Check sheet for the modelled part. Datum: model origin and axes. Units: mm. Coordinates: 2 decimals unless noted, no trailing zeros. Order: outer loops, then holes, each group sorted by start corner. A loop starts at its lowest first (then second) coordinate and runs counter-clockwise, first axis right, second up.
from build123d import *

# Parameters (mm, degrees)
SKETCH1_R           = 1.5
BOSS_EXTRUDE1_DEPTH = 3.18
SKETCH2_R           = 10
CUT_EXTRUDE1_DEPTH  = 3.18


with BuildPart() as part:
    # Sketch1 → Boss-Extrude1 (new body)
    with BuildSketch(Plane(origin=(0, 0, 0), x_dir=(1, 0, 0), z_dir=(0, 1, 0))):
        with BuildLine():
            Line((-36.950288588, 11.035836474), (7.707885855, 14.942920471))
            ThreePointArc((7.707885855, 14.942920471), (24.015221996, 0), (7.707885855, -14.942920471))
            Line((7.707885855, -14.942920471), (-36.950288588, -11.035836474))
            ThreePointArc((-36.950288588, -11.035836474), (-47.062769581, 0), (-36.950288588, 11.035836474))
        make_face()
        with Locations(Location((-35.984778004, 0, 0), (0, 0, 90))):
            Circle(SKETCH1_R, mode=Mode.SUBTRACT)
    extrude(amount=BOSS_EXTRUDE1_DEPTH)

    # Sketch2 → Cut-Extrude1 (cut)
    with BuildSketch(Plane.XZ):
        with Locations(Location((7.707885855, 0, 0), (0, 0, 270))):
            Circle(SKETCH2_R)
    extrude(amount=-CUT_EXTRUDE1_DEPTH, mode=Mode.SUBTRACT)


solid = part.part
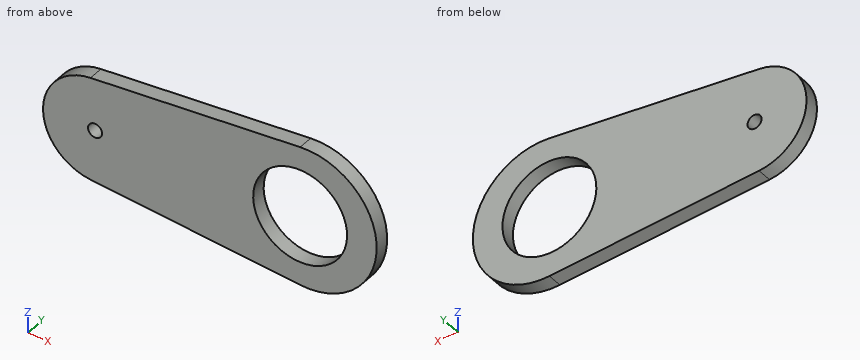
(1) Cross-section at B-B (z = -3.5). Enter the section's corners in (x, y), and give its area (3 significant figures).
Filled in:
outline: (-46.5, 0) - (-1.66, 0) - (-1.66, 3.18) - (-46.5, 3.18) - close; (17.08, 0) - (23.6, 0) - (23.6, 3.18) - (17.08, 3.18) - close
area: 163 mm2
(2) Thickness scan on probe 1 along X at (y, z) = (1.8, 0); probe 2 along Z at (x, y) = (11, 1.05); probe 3 along Z at (x, y) = (3.5, 1.9). Record the ranges inside material, lowest first.
Filled in:
probe 1: x = -47.06 to -37.48, -34.48 to -2.29, 17.71 to 24.02
probe 2: z = -14.87 to -9.44, 9.44 to 14.87
probe 3: z = -14.57 to -9.07, 9.07 to 14.57
(3) Cross-section at C-C (y = 2.05). Enter the section's corners in (x, z), and give its area (3 significant figures).
Filled in:
outline: (-36.95, -11.04) - (7.71, -14.94) arc R15 ccw (long way) to (7.71, 14.94) - (-36.95, 11.04) arc R11.08 ccw to start; hole circle Ø3 at (-35.98, 0); hole circle Ø20 at (7.71, 0)
area: 1,400 mm2
(4) Cross-section at A-A (z = 0). Enter the section's corners in (x, y), and give its area (3 significant figures).
Filled in:
outline: (-47.06, 0) - (-37.48, 0) - (-37.48, 3.18) - (-47.06, 3.18) - close; (-34.48, 0) - (-2.29, 0) - (-2.29, 3.18) - (-34.48, 3.18) - close; (17.71, 0) - (24.02, 0) - (24.02, 3.18) - (17.71, 3.18) - close
area: 153 mm2
(5) Go/stop test with flat-tipped pins: P1, Ø1.5, axis at y = 2, z = 1.5, coming from the +X side; P2, Ø10, axis at x = 3.5, z = 2, coming from the +Y side; P3, Ø1, axis at x = -29.5, y = 2.5, coming from the -Z side. Record where each tip stops, or that it passes through.
Filled in:
P1: stops at x = 24
P2: passes through
P3: stops at z = -11.73
(6) Cross-section at D-D (z = -7). Enter the section's corners in (x, y).
Filled in:
outline: (-44.57, 0) - (0.57, 0) - (0.57, 3.18) - (-44.57, 3.18) - close; (14.85, 0) - (22.28, 0) - (22.28, 3.18) - (14.85, 3.18) - close
